Autodesk Inventor part; units mm, degrees
ref_plane "YZ Plane" through (0, 0, 0) normal (1, 0, 0) x (0, 1, 0)
ref_plane "XZ Plane" through (0, 0, 0) normal (0, 1, 0) x (-1, 0, 0)
ref_plane "XY Plane" through (0, 0, 0) normal (0, 0, 1) x (1, 0, 0)
sketch "Sketch66" plane through (0, 0, 0) normal (0, 0, 1) x (1, 0, 0)
  line L0 (-120, -39.5) -> (120, -39.5)
  line L1 (120, -39.5) -> (120, 39.5)
  line L2 (120, 39.5) -> (-120, 39.5)
  line L3 (-120, 39.5) -> (-120, -39.5)
  line L4 (-120, -39.5) -> (120, 39.5) construction
  line L5 (120, -39.5) -> (-120, 39.5) construction
  point P0 (0, 0)
  dimension "d179" = 240
  dimension "d180" = 79
extrude "Extrusion45" add sketch "Sketch66" along normal blind 3
sketch "Sketch68" plane through (0, 0, 3) normal (0, 0, 1) x (1, 0, 0)
  circle A0 centre (-112, 31.5) radius 3.5
  circle A1 centre (-112, -31.5) radius 3.5
  circle A2 centre (112, 31.5) radius 3.5
  circle A3 centre (112, -31.5) radius 3.5
  point P0 (0, 0)
  dimension "d186" = 7
  dimension "d187" = 7
  dimension "d188" = 7
  dimension "d189" = 7
extrude "Extrusion47" cut sketch "Sketch68" against normal through all
sketch "Sketch69" plane through (0, 0, 3) normal (0, 0, 1) x (1, 0, 0)
  circle A0 centre (-27, -23.5) radius 3.5
  circle A1 centre (27, -23.5) radius 3.5
  point P0 (0, 0)
  dimension "d192" = 7
  dimension "d193" = 7
extrude "Extrusion48" cut sketch "Sketch69" against normal through all
equation "\"d187\" = d186"
equation "\"d188\" = d186"
equation "\"d189\" = d186"
equation "\"d192\" = d186"
equation "\"d193\" = d186"
properties part number "magnet_test_print_v02"
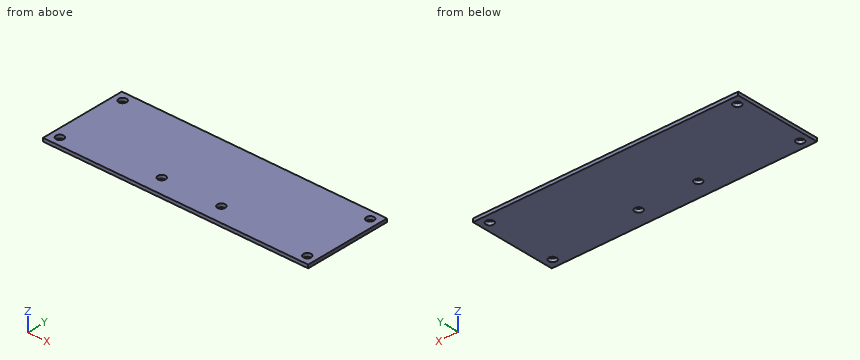
Model file for the job. Use its own axes, mm. Give positions to 0.01 mm unless a question says otherwise; leave off trailing zeros. Loops run counter-clockwise (first coordinate to the right, second up) from the corner with the lowest first, then second, coordinate; pieces in that order, holes last. Notation, with made-up numbers: M 33.25,32 L 43.25,32 A31 ccw 43.25,59 Z; hole C -8,-38.5 d9. An arc over 180 degrees is marked long. Use one line per item in the form item = value.
Item 1: Slice it at B-B on y = -23.5. List the corners of the cut face in (x, z), and give its area (3 significant figures).
Filled in:
outline = M -120,0 L -30.5,0 L -30.5,3 L -120,3 Z; M -23.5,0 L 23.5,0 L 23.5,3 L -23.5,3 Z; M 30.5,0 L 120,0 L 120,3 L 30.5,3 Z
area = 678 mm^2
Item 2: Drill centre lines: L1, parallel to Y at x = 112, z = 0.6; L2, parallel to Y at x = -27, z = 0.6; L3, parallel to X at y = 32.5, z = 0.6. Where is each one in solid material? Low to high.
Filled in:
L1 = -39.5 to -35, -28 to 28, 35 to 39.5
L2 = -39.5 to -27, -20 to 39.5
L3 = -120 to -115.35, -108.65 to 108.65, 115.35 to 120
Item 3: Slice it at C-C on x = -112. List the corners of the cut face in (y, z).
Filled in:
outline = M -39.5,0 L -35,0 L -35,3 L -39.5,3 Z; M -28,0 L 28,0 L 28,3 L -28,3 Z; M 35,0 L 39.5,0 L 39.5,3 L 35,3 Z
Item 4: Slice it at A-A on x = -27. List the corners of the cut face in (y, z), and give its area (3 significant figures).
Filled in:
outline = M -39.5,0 L -27,0 L -27,3 L -39.5,3 Z; M -20,0 L 39.5,0 L 39.5,3 L -20,3 Z
area = 216 mm^2
Item 5: Flat gauge pins, fed straight in: pin 1 Ø11 at (x, y) = (-112, -31.5) entering from -Z; pin 2 Ø6.5 at (x, y) = (-27, -23.5) entering from +Z. Where does each tip first touch, or does it go through?
Filled in:
pin_1 = 0
pin_2 = through
